Source: CAD feature listing. Evaluate the final solid. Frame: model axes, mm. Face numbers are marked on the shaded views. A direction names the side the tool comes from. Coordinates: 2 decimals unless noted, no trailing zeros. Order: outer loops, then holes, each group sorted by start corner. A loop starts at its lowest first (then second) coordinate and runs counter-clockwise, first axis right, second up.
Item 1: Mould query, pull axis X, two halves, no side actions, for the marked faces 1, 2, 3 and 4. Classes: released by +X, released by -X, zero draft, split by the parting line, or undercut.
Item 2: Section C-C on z = 12.5. Return the cut outline in (x, y).
Item 3: Contact query for flat-ended pins moving along their axis: P1, Ø10.5, axis at y = -56.5, z = 16, coming from the -X side; P2, Ø10, axis at x = 47.5, z = 19.5, coming from the +Y side; P3, Ø5, axis at x = 79, z = 4.5, coming from the -Y side; P4, Ø5, axis at x = 20, y = 17.5, coming from the +Z side. Output: stop coordinate, or through.
Item 4: Section B-B on x = 6.5. Return the cut outline in (y, z).
Item 5: Section D-D on y = 10. Return the cut outline in (x, z).
Item 6: Ray query, line 1 (Y direction, x = -52.5, z = 17.5); line 2 (X direction, y = -31.5, z = 16); line 3 (X direction, y = -5, z = 19.5). Return the intervals inside material, ascending.
Item 7: Reachability of the marked faces 5, 6 and 7 from +Z, -Z, +X, -X, +Y, -Y: full face, straight path, thin tool, end or side. Return the list, or none.
Item 8: Section A-A on y = -20. Return the cut outline in (x, z), then the cut area to 3 significant figures.
from build123d import *

# Parameters (mm, degrees)
F1_DEPTH = 25
F2_R     = 7.5
F3_DEPTH = 25


with BuildPart() as f1:
    # F0 (on Top) → F1 (new body)
    with BuildSketch(Plane.XY):
        with BuildLine():
            Line((-18.5831710696, -64.4391401045), (0, -64.4391401045))
            Line((0, -64.4391401045), (18.5831710696, -64.4391401045))
            Line((18.5831710696, -64.4391401045), (18.5831710696, -51.1375991389))
            ThreePointArc((18.5831710696, -51.1375991389), (28.4354251443, -41.8873150264), (34.0493159096, -29.594272401))
            Line((34.0493159096, -29.594272401), (66.9053312008, -29.594272401))
            Line((66.9053312008, -29.594272401), (100, -4.7732681821))
            Line((100, -4.7732681821), (100, 29.4510790908))
            Line((100, 29.4510790908), (66.9053312008, 17.1837710472))
            Line((66.9053312008, 17.1837710472), (0, 17.1837710472))
            Line((0, 17.1837710472), (-66.9053312008, 17.1837710472))
            Line((-66.9053312008, 17.1837710472), (-100, 29.4510790908))
            Line((-100, 29.4510790908), (-100, -4.7732681821))
            Line((-100, -4.7732681821), (-66.9053312008, -29.594272401))
            Line((-66.9053312008, -29.594272401), (-34.0493159096, -29.594272401))
            ThreePointArc((-34.0493159096, -29.594272401), (-28.4354251443, -41.8873150264), (-18.5831710696, -51.1375991389))
            Line((-18.5831710696, -51.1375991389), (-18.5831710696, -64.4391401045))
        make_face()
        with BuildLine():
            ThreePointArc((0, 2.6473924518), (24.120664224, -21.4732717723), (0, -45.5939359963))
            ThreePointArc((0, -45.5939359963), (-24.120664224, -21.4732717723), (0, 2.6473924518))
        make_face(mode=Mode.SUBTRACT)
    extrude(amount=F1_DEPTH)

    # F2 (on face) → F3 (join)
    with BuildSketch(Plane(origin=(-100, 0, 0), x_dir=(0, -1, 0), z_dir=(-1, 0, 0))):
        with Locations((-12.3389054544, 12.5)):
            Circle(F2_R)
    extrude(amount=F3_DEPTH)

    # F4: F1 across plane


with BuildPart() as f1_1:
    add(f1.part)
    add(f1.part.mirror(Plane.YZ))


solid = f1_1.part
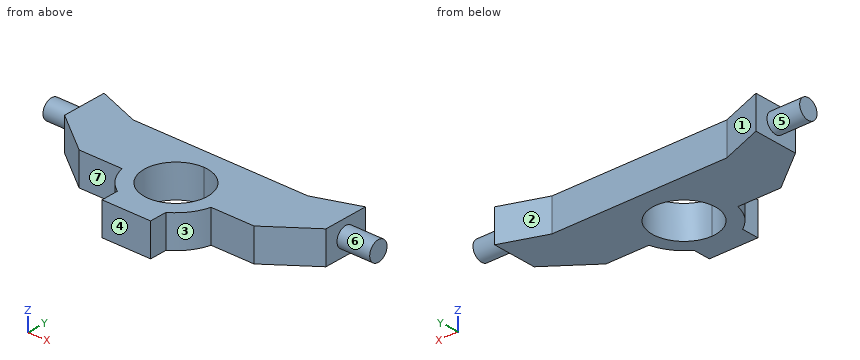
Answer list:
1. face 1: undercut
1. face 2: undercut
1. face 3: released by +X
1. face 4: zero draft
2. outline: (-125, 4.84) - (-100, 4.84) - (-100, -4.77) - (-66.91, -29.59) - (-34.05, -29.59) arc R35 ccw to (-18.58, -51.14) - (-18.58, -64.44) - (18.58, -64.44) - (18.58, -51.14) arc R35 ccw to (34.05, -29.59) - (66.91, -29.59) - (100, -4.77) - (100, 4.84) - (125, 4.84) - (125, 19.84) - (100, 19.84) - (100, 29.45) - (66.91, 17.18) - (-66.91, 17.18) - (-100, 29.45) - (-100, 19.84) - (-125, 19.84) - close; hole circle Ø48.24 at (0, -21.47)
3. P1: stops at x = -18.58
3. P2: stops at y = 17.18
3. P3: stops at y = -22.4
3. P4: stops at z = 25
4. outline: (-64.44, 0) - (-44.7, 0) - (-44.7, 25) - (-64.44, 25) - close; (1.76, 0) - (17.18, 0) - (17.18, 25) - (1.76, 25) - close
5. outline: (-125, 5.37) - (-100, 5.37) - (-100, 0) - (100, 0) - (100, 5.37) - (125, 5.37) - (125, 19.63) - (100, 19.63) - (100, 25) - (-100, 25) - (-100, 19.63) - (-125, 19.63) - close
6. line 1: y = -29.59 to 17.18
6. line 2: x = -33.54 to -21.94, 21.94 to 33.54
6. line 3: x = -99.7 to -17.62, 17.62 to 99.7
7. face 5: -X
7. face 6: +X
7. face 7: +Z, -Z, -X, -Y
8. outline: (-79.7, 0) - (-24.08, 0) - (-24.08, 25) - (-79.7, 25) - close; (24.08, 0) - (79.7, 0) - (79.7, 25) - (24.08, 25) - close
8. area: 2,780 mm2
